from build123d import *

# Parameters (mm, degrees)
SKETCH2_W           = 50
SKETCH2_H           = 90
SKETCH2_R           = 16
SKETCH2_R_2         = 2.15
BOSS_EXTRUDE1_DEPTH = 5
SKETCH3_W           = 50
SKETCH3_H           = 5
BOSS_EXTRUDE2_DEPTH = 100
SKETCH4_R           = 2.5
CUT_EXTRUDE1_DEPTH  = 134.603892159
CHAMFER1_SIZE       = 2.8


with BuildPart() as part:
    # Sketch2 → Boss-Extrude1 (new body)
    with BuildSketch(Plane.XY):
        Rectangle(SKETCH2_W, SKETCH2_H)
        with Locations((0, 13)):
            Circle(SKETCH2_R, mode=Mode.SUBTRACT)
        with Locations((-16.263455967, 29.263455967)):
            Circle(SKETCH2_R_2, mode=Mode.SUBTRACT)
        with Locations((16.263455967, 29.263455967)):
            Circle(SKETCH2_R_2, mode=Mode.SUBTRACT)
        with Locations((16.263455967, -3.263455967)):
            Circle(SKETCH2_R_2, mode=Mode.SUBTRACT)
        with Locations((-16.263455967, -3.263455967)):
            Circle(SKETCH2_R_2, mode=Mode.SUBTRACT)
    extrude(amount=BOSS_EXTRUDE1_DEPTH)

    # Sketch3 → Boss-Extrude2 (add)
    with BuildSketch(Plane(origin=(0, 0, 0), x_dir=(-1, 0, 0), z_dir=(0, 0, -1))):
        with Locations((0, -42.5)):
            Rectangle(SKETCH3_W, SKETCH3_H)
    extrude(amount=BOSS_EXTRUDE2_DEPTH)

    # Sketch4 → Cut-Extrude1 (cut, through all)
    with BuildSketch(Plane(origin=(0, -40, 0), x_dir=(1, 0, 0), z_dir=(0, 1, 0))):
        with Locations(Location((-10, 92.002293004, 0), (0, 0, 180))):
            Circle(SKETCH4_R)
        with Locations(Location((10, 92.002293004, 0), (0, 0, 180))):
            Circle(SKETCH4_R)
        with Locations(Location((-10, 12.002293004, 0), (0, 0, 180))):
            Circle(SKETCH4_R)
        with Locations(Location((10, 12.002293004, 0), (0, 0, 180))):
            Circle(SKETCH4_R)
        with Locations(Location((-10, 52.002293004, 0), (0, 0, 180))):
            Circle(SKETCH4_R)
        with Locations(Location((10, 52.002293004, 0), (0, 0, 180))):
            Circle(SKETCH4_R)
    extrude(amount=-CUT_EXTRUDE1_DEPTH, mode=Mode.SUBTRACT)

    # Chamfer1
    chamfer1_edges = [part.edges().sort_by_distance(p)[0] for p in [
        (-7.5, -40, -92.002293004),
        (12.5, -40, -92.002293004),
        (-7.5, -40, -12.002293004),
        (12.5, -40, -12.002293004),
        (-7.5, -40, -52.002293004),
        (12.5, -40, -52.002293004),
    ]]
    chamfer(chamfer1_edges, length=CHAMFER1_SIZE)


solid = part.part
Input: part model. Units: mm. Frame: model coordinates. A direction names the side the tool comes from. Coordinates: 2 decimals unless noted, no trailing zeros. Loops run counter-clockwise (first coordinate to the right, second up) from the corner with the lowest first, then second, coordinate; pieces in that order, holes last. Notation, with made-up numbers: (35, 48) -> (40, 48) arc R27 cw to (40, 81) -> close; hole circle Ø10 at (49.25, -29.75). An arc over 180 degrees is marked (long way). Write each question's results on one line, items separated by ' | '. Start each with the question number.
Q1. Section C-C, the plane x = -10. Return the cut outline in (y, z).
Q2. Ray query, line 1 (Z direction, x = 10, y = -43); line 2 (Y direction, x = 21, z = -75); line 3 (Z direction, x = 22, y = 26). Return the intervals inside material, ascending. Write a range as from..to.
Q3. Section B-B, the plane y = 13. Return the cut outline in (x, z), plus the area to 3 significant figures.
Q4. Section A-A, the plane x = 0. Return the cut outline in (y, z).
Q5. Pin query (flat end, axial travel): pin 1 (2.5 mm diameter, centred on x = -16.26, y = 29.26, fed in from -Z); pin 2 (6 mm diameter, centred on x = 10, z = -52, fed in from +Y); pin 3 (6 mm diameter, centred on x = -6, y = -30.5, fed in from -Z); pin 4 (6.5 mm diameter, centred on x = 10, z = -92, fed in from -Y). Return the tip coordinate at first contact, or that it passes through.
Q6. Reachability of faces 5 (the flat face through (0, -45, -47)), 6 (the flat face through (0, -40, -49)) from +Z, -Z, +X, -X, +Y, -Y: full face, straight path, thin tool, end or side. Return the list, or none.
Q7. Pull-direction query (Z, two-part tool) for faces 1 (the cylindrical face through (18.314, 29.909, 2.465)), 2 (the cylindrical face through (11.84, -43.88, -10.31)), 3 (the conical face through (-9.657, -42.664, -9.389)), 4 (the flat face through (0, -9, 5)); classes: released by +Z, released by -Z, zero draft, split by the parting line, or undercut.
Q8. Section D-D, the plane y = 24. Return the cut outline in (x, z), plus the area to 3 significant figures.
Found:
1) outline: (-45, -100) -> (-40, -100) -> (-40, -97.3) -> (-42.8, -94.5) -> (-45, -94.5) -> close; (-45, -89.5) -> (-42.8, -89.5) -> (-40, -86.7) -> (-40, -57.3) -> (-42.8, -54.5) -> (-45, -54.5) -> close; (-45, -49.5) -> (-42.8, -49.5) -> (-40, -46.7) -> (-40, -17.3) -> (-42.8, -14.5) -> (-45, -14.5) -> close; (-45, -9.5) -> (-42.8, -9.5) -> (-40, -6.7) -> (-40, 0) -> (0.51, 0) -> (0.51, 5) -> (-45, 5) -> close; (25.49, 0) -> (45, 0) -> (45, 5) -> (25.49, 5) -> close
2) line 1: -100..-94.5, -89.5..-54.5, -49.5..-14.5, -9.5..5 | line 2: -45..-40 | line 3: 0..5
3) outline: (-25, 0) -> (-16, 0) -> (-16, 5) -> (-25, 5) -> close; (16, 0) -> (25, 0) -> (25, 5) -> (16, 5) -> close | area: 90.0 mm2
4) outline: (-45, -100) -> (-40, -100) -> (-40, 0) -> (-3, 0) -> (-3, 5) -> (-45, 5) -> close; (29, 0) -> (45, 0) -> (45, 5) -> (29, 5) -> close
5) pin 1: through | pin 2: y = -42.3 | pin 3: z = 0 | pin 4: y = -45
6) face 5: +Z, -Z, +X, -X, -Y | face 6: -Z, +X, -X, +Y
7) face 1: zero draft | face 2: undercut | face 3: undercut | face 4: released by +Z
8) outline: (-25, 0) -> (-11.62, 0) -> (-11.62, 5) -> (-25, 5) -> close; (11.62, 0) -> (25, 0) -> (25, 5) -> (11.62, 5) -> close | area: 134 mm2
